from build123d import *

# Parameters (mm, degrees)
SKETCH1_W             = 10.6165
SKETCH1_H             = 20
SKETCH1_W_2           = 10.732
SKETCH1_H_2           = 10
BOSS_EXTRUDE1_DEPTH   = 6
SKETCH2_W             = 10.6165
SKETCH2_H             = 5
BOSS_EXTRUDE2_DEPTH   = 5
CHAMFER1_SIZE         = 2
BOSS_EXTRUDE3_START   = -10
SKETCH3_R             = 4.95
BOSS_EXTRUDE3_DEPTH   = 20
BOSS_EXTRUDE4_START   = 10
SKETCH3_3_R           = 4.95
BOSS_EXTRUDE4_DEPTH   = 10
BOSS_EXTRUDE5_START   = -20
SKETCH3_4_R           = 4.95
BOSS_EXTRUDE5_DEPTH   = 10
BOSS_EXTRUDE6_START   = -40
SKETCH3_5_R           = 4.95
BOSS_EXTRUDE6_DEPTH   = 20
BOSS_EXTRUDE7_START   = -50
SKETCH3_6_R           = 4.95
BOSS_EXTRUDE7_DEPTH   = 10
F_1_0MM_DOWEL_HOLE1_D = 2.2
CUT_EXTRUDE1_START    = -0.2
CUT_EXTRUDE1_DEPTH    = 0.2
CUT_EXTRUDE2_START    = -30.2
CUT_EXTRUDE2_DEPTH    = 10.4
CUT_EXTRUDE3_START    = -50
CUT_EXTRUDE3_DEPTH    = 0.2
SKETCH10_W            = 3
SKETCH10_H            = 49.6
BOSS_EXTRUDE8_DEPTH   = 40


with BuildPart() as part:
    # Sketch1 → Boss-Extrude1 (new body)
    with BuildSketch(Plane(origin=(0, 0, 0), x_dir=(1, 0, 0), z_dir=(0, 1, 0))):
        Polygon((16.2325, -10), (10.6165, -10), (5.5005, -10), (5.5005, -20), (16.2325, -20), align=None)
        Polygon((10.6165, 0), (0, 0), (0, -10), (5.5005, -10), (10.6165, -10), align=None)
        Polygon((0, 10), (0, 0), (10.6165, 0), (10.6165, 10), (5.5005, 10), align=None)
        Polygon((5.5005, 10), (10.6165, 10), (16.2325, 10), (16.2325, 20), (10.6165, 20), (5.5005, 20), align=None)
        with Locations((5.30825, 30)):
            Rectangle(SKETCH1_W, SKETCH1_H)
        with Locations((10.8665, 45)):
            Rectangle(SKETCH1_W_2, SKETCH1_H_2)
    extrude(amount=BOSS_EXTRUDE1_DEPTH)

    # Sketch2 → Boss-Extrude2 (add)
    with BuildSketch(Plane(origin=(0, 6, 0), x_dir=(1, 0, 0), z_dir=(0, 1, 0))):
        with Locations((5.30825, 7.5)):
            Rectangle(SKETCH2_W, SKETCH2_H)
        with Locations((5.30825, -7.5)):
            Rectangle(SKETCH2_W, SKETCH2_H)
        with Locations((5.30825, 37.5)):
            Rectangle(SKETCH2_W, SKETCH2_H)
        with Locations((5.30825, 22.5)):
            Rectangle(SKETCH2_W, SKETCH2_H)
    extrude(amount=BOSS_EXTRUDE2_DEPTH)

    # Chamfer1
    chamfer1_edges = [part.edges().sort_by_distance(p)[0] for p in [
        (5.30825, 11, -35),
        (5.30825, 11, -25),
        (5.30825, 11, -5),
        (5.30825, 11, 5),
    ]]
    chamfer(chamfer1_edges, length=CHAMFER1_SIZE)

    # Sketch3 → Boss-Extrude3 (add)
    with BuildSketch(Plane.XY.offset(BOSS_EXTRUDE3_START)):
        with Locations((0, 6.05)):
            Circle(SKETCH3_R)
    extrude(amount=BOSS_EXTRUDE3_DEPTH)

    # Sketch3<3> → Boss-Extrude4 (add)
    with BuildSketch(Plane.XY.offset(BOSS_EXTRUDE4_START)):
        with Locations((16.2325, 6.05)):
            Circle(SKETCH3_3_R)
    extrude(amount=BOSS_EXTRUDE4_DEPTH)

    # Sketch3<4> → Boss-Extrude5 (add)
    with BuildSketch(Plane.XY.offset(BOSS_EXTRUDE5_START)):
        with Locations((16.2325, 6.05)):
            Circle(SKETCH3_4_R)
    extrude(amount=BOSS_EXTRUDE5_DEPTH)

    # Sketch3<5> → Boss-Extrude6 (add)
    with BuildSketch(Plane.XY.offset(BOSS_EXTRUDE6_START)):
        with Locations((0, 6.05)):
            Circle(SKETCH3_5_R)
    extrude(amount=BOSS_EXTRUDE6_DEPTH)

    # Sketch3<6> → Boss-Extrude7 (add)
    with BuildSketch(Plane.XY.offset(BOSS_EXTRUDE7_START)):
        with Locations((16.2325, 6.05)):
            Circle(SKETCH3_6_R)
    extrude(amount=BOSS_EXTRUDE7_DEPTH)

    # Ø1.0mm Dowel Hole1 (through all)
    with Locations(Plane.XY.offset(20)):
        with Locations((0, 6.05), (16.2325, 6.05)):
            Hole(F_1_0MM_DOWEL_HOLE1_D / 2)

    # Sketch9 → Cut-Extrude1 (cut)
    with BuildSketch(Plane.XY.offset(10).offset(CUT_EXTRUDE1_START)):
        with BuildLine():
            Line((5.5005, 6), (5.5005, 11))
            Line((5.5005, 11), (0, 11))
            ThreePointArc((0, 11), (-4.95, 6.05), (0, 1.1))
            Line((0, 1.1), (0, 0))
            Line((0, 0), (5.5005, 0))
            Line((5.5005, 0), (5.5005, 6))
        make_face()
    extrude(amount=CUT_EXTRUDE1_DEPTH, mode=Mode.SUBTRACT)

    # Sketch9<2> → Cut-Extrude2 (cut)
    with BuildSketch(Plane.XY.offset(10).offset(CUT_EXTRUDE2_START)):
        with BuildLine():
            Line((5.5005, 0), (5.5005, 6))
            Line((5.5005, 6), (5.5005, 11))
            Line((5.5005, 11), (0, 11))
            ThreePointArc((0, 11), (-4.95, 6.05), (0, 1.1))
            Line((0, 1.1), (0, 0))
            Line((0, 0), (5.5005, 0))
        make_face()
    extrude(amount=CUT_EXTRUDE2_DEPTH, mode=Mode.SUBTRACT)

    # Sketch9<4> → Cut-Extrude3 (cut)
    with BuildSketch(Plane.XY.offset(10).offset(CUT_EXTRUDE3_START)):
        with BuildLine():
            Line((5.5005, 0), (5.5005, 6))
            Line((5.5005, 6), (5.5005, 11))
            Line((5.5005, 11), (0, 11))
            ThreePointArc((0, 11), (-4.95, 6.05), (0, 1.1))
            Line((0, 1.1), (0, 0))
            Line((0, 0), (5.5005, 0))
        make_face()
    extrude(amount=CUT_EXTRUDE3_DEPTH, mode=Mode.SUBTRACT)

    # Sketch10 → Boss-Extrude8 (add)
    with BuildSketch(Plane.XZ):
        with Locations((8.11625, -15)):
            Rectangle(SKETCH10_W, SKETCH10_H)
    extrude(amount=BOSS_EXTRUDE8_DEPTH)


solid = part.part
Input: part model. Units: mm. Frame: model coordinates. A direction names the side the tool comes from. Coordinates: 2 decimals unless noted, no trailing zeros. Loops run counter-clockwise (first coordinate to the right, second up) from the corner with the lowest first, then second, coordinate; pieces in that order, holes last.
Q1. Contact query for flat-ended pins moving along their axis: pin 1 (10 mm diameter, centred on y = -5.5, z = -3, fed in from +X); pin 2 (1.5 mm diameter, centred on y = 4.5, z = -2, fed in from +X); pin 3 (8.5 mm diameter, centred on x = -1, y = 3.5, fed in from +Z); pin 4 (1.8 mm diameter, centred on x = 16.23, y = 6.05, fed in from +Z). Output: stop coordinate, or through.
Q2. Cut plane B-B (x = 7.75). Output: boundary loops of the cut face in (y, z), then the cut area to 3 significant figures.
Q3. Cut plane A-A (z = -3.5). Output: boundary loops of the cut face in (x, y).
Q4. Cut plane C-C (y = 2.5). Output: boundary loops of the cut face in (x, z).
Q5. Draft query along Z for faces 4 (the face through (6, 10, -6)), 5 (the face through (15.216, 5.629, -15.07)), 6 (the face through (13, 4, -50)). Return one class per face: +Z half, -Z half, draft (parallel to the pull), parting line (faces both ways), or undercut.
Q6. Cut plane D-D (x = -2). Output: boundary loops of the cut face in (y, z).
Q7. Material intervals for line 1 (Z direction, x = -2.5, y = 3); line 2 (X direction, y = -21.5, z = -19.5); line 3 (Z direction, x = 9.5, y = -11.5), sorted ascending.
Q8. Set-up query: faces 1 (the face through (1.4, 5.6, -20.2)), 2 (the face through (8, 6, 15)), 3 (the face through (-4.73, 7.51, -0.14)). Return all of +Z, -Z, +X, -X, +Y, -Y with unobstructed straight access to the full face (end or side cutting, diameter ignored); none if empty.
Working result:
1. pin 1: stops at x = 9.62
1. pin 2: stops at x = 10.62
1. pin 3: stops at z = 9.8
1. pin 4: passes through
2. outline: (-40, -39.8) - (0, -39.8) - (0, -50) - (6, -50) - (6, -40) - (11, -40) - (11, -37) - (9, -35) - (6, -35) - (6, -25) - (9, -25) - (11, -23) - (11, -20) - (6, -20) - (6, -10) - (11, -10) - (11, -7) - (9, -5) - (6, -5) - (6, 5) - (9, 5) - (11, 7) - (11, 10) - (6, 10) - (6, 20) - (0, 20) - (0, 9.8) - (-40, 9.8) - close
2. area: 2,500 mm2
3. outline: (0, 0) - (6.62, 0) - (6.62, -40) - (9.62, -40) - (9.62, 0) - (10.62, 0) - (10.62, 6) - (4.95, 6) arc R4.95 ccw (long way) to (0, 1.1) - close; hole circle Ø2.2 at (0, 6.05)
4. outline: (-3.45, -39.8) - (5.5, -39.8) - (5.5, -50) - (19.68, -50) - (19.68, -40) - (10.62, -40) - (10.62, -20) - (19.68, -20) - (19.68, -10) - (10.62, -10) - (10.62, 10) - (19.68, 10) - (19.68, 20) - (5.5, 20) - (5.5, 9.8) - (-3.45, 9.8) - (-3.45, -9.8) - (5.5, -9.8) - (5.5, -20.2) - (-3.45, -20.2) - close
5. face 4: undercut
5. face 5: draft
5. face 6: -Z half
6. outline: (1.52, -39.8) - (10.58, -39.8) - (10.58, -20.2) - (1.52, -20.2) - close; (1.52, -9.8) - (10.58, -9.8) - (10.58, 9.8) - (1.52, 9.8) - close
7. line 1: z = -39.8 to -20.2, -9.8 to 9.8
7. line 2: x = 6.62 to 9.62
7. line 3: z = -39.8 to 9.8
8. face 1: -X, +Y, -Y
8. face 2: +Z, -X, +Y
8. face 3: none
